Design review of the part shown in the three views and the two pictorial views. Dimensions are in mm from the part's minimum x, y and z. A direction names the side the tool comes from. Round coordinates to 2 decimals unless told otherwise and drop trailing zeros. Write each loop counter-clockwise with the first axis right and the second up, starting at its lowest first coordinate (ties: lowest second). Pieces come first, ordered by that corner, then holes. Notation, with made-up numbers: (54, -34) - (112, -34) arc R26 ccw to (112, -5) - close; hole circle Ø8 at (19.25, -21). An arc over 180 degrees is marked (long way). One line per item, written item: value. Start each with the question number.
Q1. Add section A-A on x = 10. Write out the cut boundary in (y, z), and give its area (3 significant figures).
Q2. Tool access review of the marked faces 4 and 5: name each direction out of +Z, -Z, +X, -X, +Y, -Y from which nothing blocks a thin tool from reaching the whole face with its end or side.
Q3. Clearance check with flat-ended pins moving along their axes: pin 1 Ø4 at (x, z) = (3.5, 17) entering from +Y; pin 2 Ø1 at (x, z) = (8.5, 11.5) entering from +Y; pin 3 Ø8 at (x, z) = (14.5, 20.5) entering from +Y; pin 4 Ø5 at (x, y) = (17.5, 4.5) entering from -Z. State where each tip first meets the part, or that it passes through.
Q4. Add section D-D on x = 14.25. Write out the cut boundary in (y, z), and give its area (3 significant figures).
Q5. Mouldability with a two-part tool opening along Y and no side actions: class the marked faces 1, 2 and 3 as +Y half, -Y half, draft (parallel to the pull), parting line (faces both ways), or undercut.
Q6. Add section B-B on z = 17. Write out the cut boundary in (x, y), and give its area (3 significant figures).
Q7. For probe 1 along Y at (x, z) = (10, 15.25); probe 2 along Y at (x, z) = (12.75, 11); probe 3 along Z at (x, y) = (14.25, 11.5), list the stretches that pass through material, from the lowest coordinate up.
Q8. Add section C-C on y = 11.75. Write out the cut boundary in (x, z), and give its area (3 significant figures).
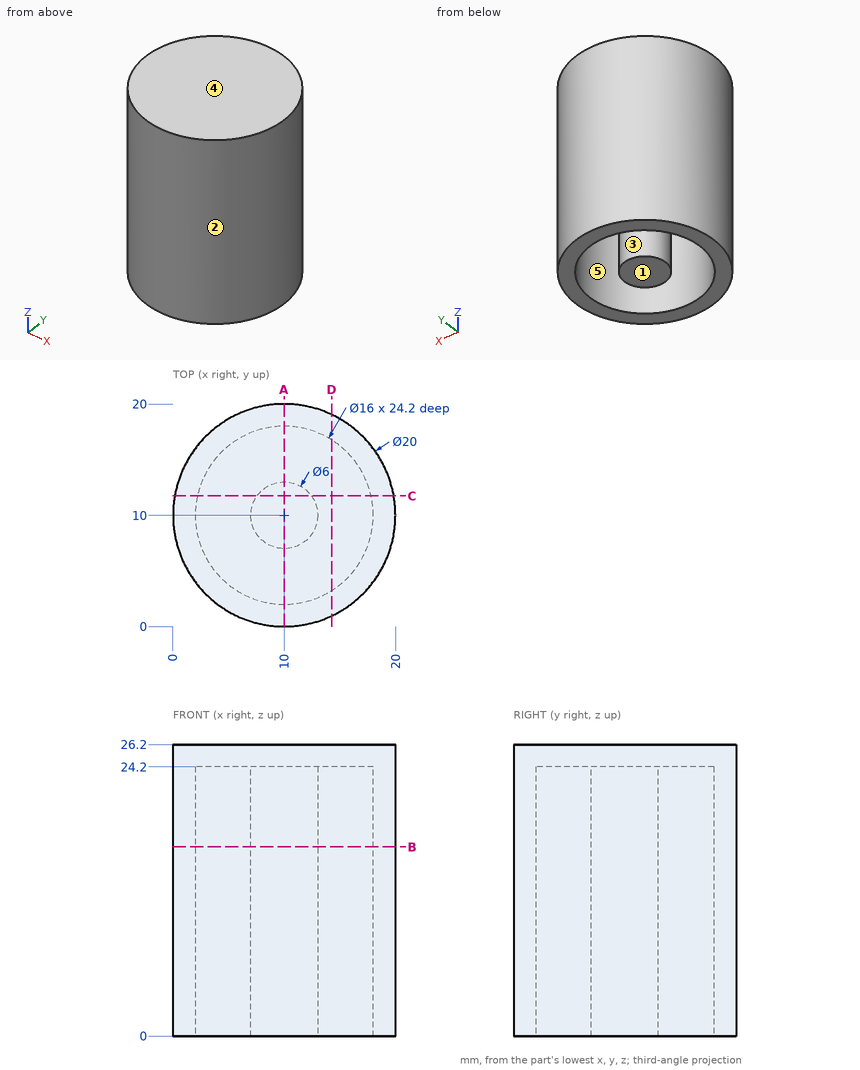
Result set:
1. outline: (0, 0) - (2, 0) - (2, 24.2) - (7, 24.2) - (7, 0) - (13, 0) - (13, 24.2) - (18, 24.2) - (18, 0) - (20, 0) - (20, 26.2) - (0, 26.2) - close
1. area: 282 mm^2
2. face 4: +Z, +X, -X, +Y, -Y
2. face 5: -Z
3. pin 1: stops at y = 18.93
3. pin 2: stops at y = 19.95
3. pin 3: stops at y = 19.99
3. pin 4: stops at z = 0
4. outline: (0.95, 0) - (3.22, 0) - (3.22, 24.2) - (16.78, 24.2) - (16.78, 0) - (19.05, 0) - (19.05, 26.2) - (0.95, 26.2) - close
4. area: 146 mm^2
5. face 1: draft
5. face 2: parting line
5. face 3: undercut
6. outline: circle Ø20 at (10, 10); circle Ø6 at (10, 10); hole circle Ø16 at (10, 10)
6. area: 141 mm^2
7. probe 1: y = 0 to 2, 7 to 13, 18 to 20
7. probe 2: y = 0.39 to 2.49, 8.8 to 11.2, 17.51 to 19.61
7. probe 3: z = 24.2 to 26.2
8. outline: (0.15, 0) - (2.19, 0) - (2.19, 24.2) - (7.56, 24.2) - (7.56, 0) - (12.44, 0) - (12.44, 24.2) - (17.81, 24.2) - (17.81, 0) - (19.85, 0) - (19.85, 26.2) - (0.15, 26.2) - close
8. area: 256 mm^2
